Part model, mm, in its own coordinate system. A direction names the side the tool comes from. Coordinates: 2 decimals unless noted, no trailing zeros. Loops run counter-clockwise (first coordinate to the right, second up) from the corner with the lowest first, then second, coordinate; pieces in that order, holes last. Notation, with made-up numbers: (-27.75, 0.5) - (-17.75, 0.5) arc R18 ccw to (-17.75, 11.5) - close; hole circle Ø5 at (86.25, 36). An arc over 180 degrees is marked (long way). Use a Markdown table: item, result. Add a question column.
1. Pull direction X, two halves, no side cores. Call faces 1 (the flat face through (0, -5, 44.5)), 2 (the conical face through (-2.63, -11.86, 52.85)), 3 (the flat face through (2, -8, 53)): pulls with the +X half, pulls with the -X half, needs draft (parallel to the pull), parting line crosses it, or undercut.
2. Wall check: probe 1 along X at (y, z) = (0.25, 21.5); probe 2 along Y at (x, z) = (0, 43.3); probe 3 along Y at (x, z) = (0, 50.5). Give the ranges that are in metal, low to high. Write a range as [from, to].
3. Band-saw the part on C-C, the plane z = 23.5. Give the cut face in (x, y), plus the area to 3 significant figures.
4. Drop flat-ended pins along their axis: pin 1 (5 mm diameter, centred on x = -4, z = 6, fed in from +Y); pin 2 (6 mm diameter, centred on y = -6.5, z = 11.5, fed in from +X); pin 3 (4 mm diameter, centred on x = -11.5, z = 45.5, fed in from -Y). Give the stop position or say it passes through.
5. 3-axis set-ups, long thin cutter, end or side, ignore diameter. For faces 4 (the cylindrical face through (-0.59, 4.46, 43.24)), 5 (the cylindrical face through (-1.73, -7.81, 19.97)), 6 (the cylindrical face through (-7.493, 0.33, 48.444)): which of +Z, -Z, +X, -X, +Y, -Y reach the whole face in a straight line?
6. Band-saw the part on A-A, the plane y = 0. Give the cut face in (x, z).
from build123d import *

# Parameters (mm, degrees)
F2_SIZE = 3
F3_SIZE = 0.5


with BuildPart() as f1:
    # F0 (on Front) → F1 (revolve)
    with BuildSketch(Plane.XZ):
        Polygon((8, 40), (8, 0), (15, 0), (15, 53), (7.5, 53), (7.5, 44.5), (4.5, 44.5), (4.5, 42.020726), align=None)
    revolve(axis=Axis((0, 0, 33.144991), (0, 0, 1)))

    # F2
    f2_edges = [f1.edges().sort_by_distance(p)[0] for p in [
        (-15, 0, 53),
    ]]
    chamfer(f2_edges, length=F2_SIZE)

    # F3
    f3_edges = [f1.edges().sort_by_distance(p)[0] for p in [
        (-7.5, 0, 53),
        (-15, 0, 0),
        (-8, 0, 0),
    ]]
    chamfer(f3_edges, length=F3_SIZE)


solid = f1.part
Geometry check:
| question | item | result |
|---|---|---|
| 1 | face 1 | undercut |
| 1 | face 2 | parting line crosses it |
| 1 | face 3 | needs draft |
| 2 | probe 1 | x = [-15, -8], [8, 15] |
| 2 | probe 2 | y = [-15, -4.5], [4.5, 15] |
| 2 | probe 3 | y = [-14.5, -7.5], [7.5, 14.5] |
| 3 | outline | circle Ø30 at (0, 0); hole circle Ø16 at (0, 0) |
| 3 | area | 506 mm^2 |
| 4 | pin 1 | stops at y = 14.92 |
| 4 | pin 2 | stops at x = 14.59 |
| 4 | pin 3 | stops at y = -11.61 |
| 5 | face 4 | +Z, -Z |
| 5 | face 5 | -Z |
| 5 | face 6 | +Z |
| 6 | outline | (-15, 0.5) - (-14.5, 0) - (-8.5, 0) - (-8, 0.5) - (-8, 40) - (-4.5, 42.02) - (-4.5, 44.5) - (-7.5, 44.5) - (-7.5, 52.5) - (-8, 53) - (-12, 53) - (-15, 50) - close; (4.5, 42.02) - (8, 40) - (8, 0.5) - (8.5, 0) - (14.5, 0) - (15, 0.5) - (15, 50) - (12, 53) - (8, 53) - (7.5, 52.5) - (7.5, 44.5) - (4.5, 44.5) - close |
